Input: dimensioned drawing with shaded views. Units: mm. Origin: part minimum x, y, z. A direction names the side the tool comes from. Round coordinates to 2 decimals unless told otherwise and drop trailing zeros. Loops run counter-clockwise (first coordinate to the right, second up) from the corner with the lowest first, then second, coordinate; pieces in that order, holes last. Notation, with made-up numbers: (58, 51.5) - (109, 51.5) arc R4 cw to (109, 58.5) - close; hole circle Ø10 at (54, 82). An arc over 180 degrees is marked (long way). Answer as CSV lines item,"result".
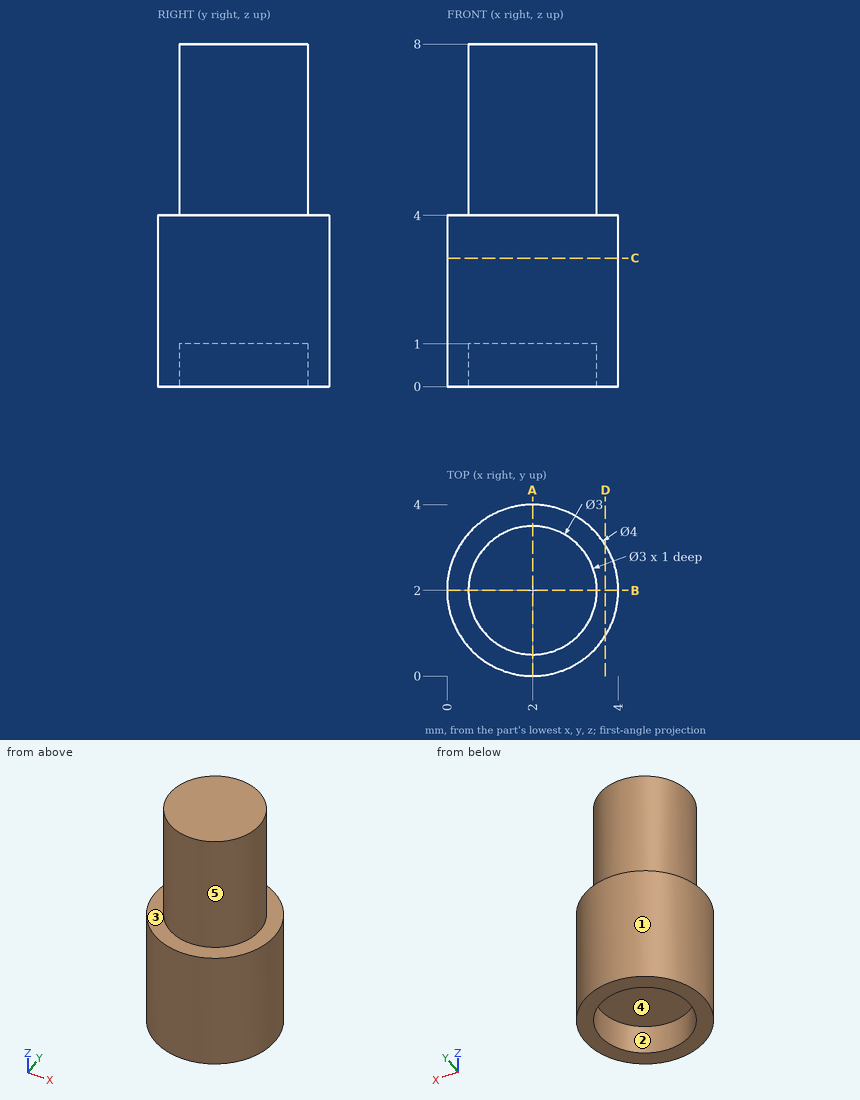
(1) Pin query (flat end, axial travel): P1, Ø1.5, axis at x = 2, y = 2.5, coming from the -Z side. Return the tip coordinate at first contact, or that it passes through.
Findings below:
P1,"z = 1"
(2) Material intervals for line 1 along Y through (x, z) = (2, 0.3); line 2 along Z through (x, y) = (3.25, 2.5); line 3 along Y through (x, z) = (2.1, 2), sorted ascending.
Findings below:
line 1,"0 to 0.5, 3.5 to 4"
line 2,"1 to 8"
line 3,"0 to 4"
(3) Section D-D (x = 3.7). Output: boundary loops of the cut face in (y, z).
Findings below:
outline,"(0.95, 0) - (3.05, 0) - (3.05, 4) - (0.95, 4) - close"
(4) Section C-C (z = 3). Output: boundary loops of the cut face in (x, y).
Findings below:
outline,"circle Ø4 at (2, 2)"
(5) Access query for the marked faces 1 and 2. Directions: +Z, -Z, +X, -X, +Y, -Y. A direction counts if a zero-diameter tool reaches every point of the face in a straight line with its end or side. Return the directions, or none.
Findings below:
face 1,"+Z, -Z"
face 2,"-Z"
(6) Draft query along Y for the marked faces 3, 4 and 5. Return one class per face: pulls with the +Y half, pulls with the -Y half, needs draft (parallel to the pull), parting line crosses it, or undercut.
Findings below:
face 3,"needs draft"
face 4,"undercut"
face 5,"parting line crosses it"
(7) Section A-A (x = 2). Output: boundary loops of the cut face in (y, z), and give its area (3 significant figures).
Findings below:
outline,"(0, 0) - (0.5, 0) - (0.5, 1) - (3.5, 1) - (3.5, 0) - (4, 0) - (4, 4) - (3.5, 4) - (3.5, 8) - (0.5, 8) - (0.5, 4) - (0, 4) - close"
area,"25.0 mm2"
